Design review of the part built by this model. Coordinates are the model's own, in mm. Coordinates: 2 decimals unless noted, no trailing zeros. Write each loop counter-clockwise with the first axis right and the second up, starting at its lowest first coordinate (ties: lowest second). Pieces come first, ordered by that corner, then holes. Notation, with made-up numbers: (58, 66.5) - (93, 66.5) arc R9 cw to (93, 75.5) - close; hole circle Ø10 at (-18, 11). An arc over 180 degrees is marked (long way). Answer as a JSON object with one key per item and string values.
```python
from build123d import *

# Parameters (mm, degrees)
BOSS_EXTRUDE1_DEPTH = 1.59
SKETCH6_R           = 1.55
CUT_EXTRUDE3_DEPTH  = 48.669302491
LPATTERN3_COUNT     = 3
LPATTERN3_PITCH     = 30
BOSS_EXTRUDE2_DEPTH = 1.59
SKETCH11_R          = 1.55
CUT_EXTRUDE7_DEPTH  = 57.396830198
SKETCH31_R          = 1.55
CUT_EXTRUDE14_DEPTH = 57.396830198


with BuildPart() as part:
    # Sketch1 → Boss-Extrude1 (new, symmetric)
    with BuildSketch(Plane.XY):
        with BuildLine():
            Line((-34.977997181, 10), (45.412002819, 10))
            ThreePointArc((45.412002819, 10), (46.5, 0), (45.412002819, -10))
            Line((45.412002819, -10), (-34.977997181, -10))
            ThreePointArc((-34.977997181, -10), (-44.977997181, 0), (-34.977997181, 10))
        make_face()
    extrude(amount=BOSS_EXTRUDE1_DEPTH, both=True)

    # Sketch6 → Cut-Extrude3 (cut, symmetric)
    with BuildSketch(Plane(origin=(0, 0, -1.59), x_dir=(-1, 0, 0), z_dir=(0, 0, -1))):
        with Locations((-12.8, 0)):
            Circle(SKETCH6_R)
    cut_extrude3 = extrude(amount=CUT_EXTRUDE3_DEPTH, both=True, mode=Mode.SUBTRACT)

    # LPattern3: Cut-Extrude3 ×3
    with Locations(*[(-i * LPATTERN3_PITCH, 0, 0) for i in range(1, LPATTERN3_COUNT)]):
        add(cut_extrude3, mode=Mode.SUBTRACT)

    # Sketch22 → Boss-Extrude2 (add, symmetric)
    with BuildSketch(Plane.XY):
        with BuildLine():
            ThreePointArc((45.412002819, -10), (46.5, 0), (45.412002819, 10))
            ThreePointArc((45.412002819, 10), (55.412002819, 0), (45.412002819, -10))
        make_face()
    extrude(amount=BOSS_EXTRUDE2_DEPTH, both=True)

    # Sketch11 → Cut-Extrude7 (cut, through all)
    with BuildSketch(Plane.XY.offset(1.59)):
        with Locations((-96.957997181, 0)):
            Circle(SKETCH11_R)
        with Locations((45.412002819, 0)):
            Circle(SKETCH11_R)
    extrude(amount=-CUT_EXTRUDE7_DEPTH, mode=Mode.SUBTRACT)

    # Sketch31 → Cut-Extrude14 (cut, through all)
    with BuildSketch(Plane.XY.offset(1.59)):
        with Locations((-34.977997181, 0)):
            Circle(SKETCH31_R)
    extrude(amount=-CUT_EXTRUDE14_DEPTH, mode=Mode.SUBTRACT)


solid = part.part
```
(1) To check wall thickness, follow line 1 (Y direction, x = -17.2, z = 0.1); line 2 (X direction, y = 0.75, z = -0.35); line 3 (X direction, y = -3.25, z = -0.95). State the ranges of each line that lie inside material, in increasing order. Write a range as from..to.
Solved:
{"line 1": "y = -10..-1.55, 1.55..10", "line 2": "x = -44.95..-36.33, -33.62..-18.56, -15.84..11.44, 14.16..44.06, 46.77..55.38", "line 3": "x = -44.44..54.87"}
(2) Take a section at B-B, the plane z = 1.1. Write out the cut boundary in (x, y).
Solved:
{"outline": "(-34.98, -10) - (45.41, -10) arc R10 ccw to (45.41, 10) - (-34.98, 10) arc R10 ccw to start; hole circle Ø3.1 at (-34.98, 0); hole circle Ø3.1 at (-17.2, 0); hole circle Ø3.1 at (12.8, 0); hole circle Ø3.1 at (45.41, 0)"}
(3) Take a section at D-D, the plane y = -7. Write out the cut boundary in (x, z).
Solved:
{"outline": "(-42.12, -1.59) - (52.55, -1.59) - (52.55, 1.59) - (-42.12, 1.59) - close"}
(4) The part is to be moulded in two halves that separate along X. For faces 1 (the face through (5, 10, 0)), 2 (the face through (11.322, 0.466, -0.022)), 3 (the face through (-44.976, -0.22, 0.022)), say which applies: pulls with the +X half, pulls with the -X half, needs draft (parallel to the pull), parting line crosses it, or undercut.
Solved:
{"face 1": "needs draft", "face 2": "undercut", "face 3": "pulls with the -X half"}
(5) Take a section at C-C, the plane x = -37.5. Write out the cut boundary in (y, z).
Solved:
{"outline": "(-9.68, -1.59) - (9.68, -1.59) - (9.68, 1.59) - (-9.68, 1.59) - close"}
(6) Take a section at A-A, the plane x = -17.2. Write out the cut boundary in (y, z).
Solved:
{"outline": "(-10, -1.59) - (-1.55, -1.59) - (-1.55, 1.59) - (-10, 1.59) - close; (1.55, -1.59) - (10, -1.59) - (10, 1.59) - (1.55, 1.59) - close"}
